CAD build for the part. Positions are in the model's coordinates, mm. A direction names the side the tool comes from. Give positions to 0.01 mm unless a question says otherwise; leave off trailing zeros. Loops run counter-clockwise (first coordinate to the right, second up) from the corner with the lowest first, then second, coordinate; pieces in that order, holes last.
Item 1: Probe probe 1 along X at (y, z) = (-4, -3); probe 2 along Z at (x, y) = (0, -1.85); probe 3 along Y at (x, z) = (11, -20). List the from-to ranges inside material, lowest first.
Item 2: Saw through at C-C on x = 7. Give the cut face in (y, z), plus the area to 3 significant figures.
Item 3: Which spindle directions (+Z, -Z, +X, -X, +Y, -Y) get a long thin tool onto all of the face, cutting with end or side? Do faces 4 (the cylindrical face through (0.31, -0.57, -21.9)), 5 (the flat face through (0, -2.5, -7)). Say none if no direction does.
Item 4: Saw through at A-A on z = -2.5. Give the cut face in (x, y).
Item 5: Drop flat-ended pins along their axis: P1, Ø8, axis at x = 10, z = 2.5, coming from the -Y side; P2, Ø1.5, axis at x = 15, y = -3, coming from the -Z side; P3, Ø0.8, axis at x = 4, y = -4, coming from the -Z side. Give the stop position or say it passes through.
Item 6: Mould opens along X. For faces 1 (the flat face through (-22.5, -3, -5)), 2 (the cylindrical face through (-4.296, -1.268, 0.189)), 3 (the flat face through (-0.31, -2.15, -22.5)) say: released by +X, released by -X, zero draft, split by the parting line, or undercut.
Item 7: Saw through at D-D on z = -12.5. Give the cut face in (x, y).
Item 8: Saw through at B-B on y = -3.25. Give the cut face in (x, z), plus the area to 3 significant figures.
from build123d import *

# Parameters (mm, degrees)
F0_W     = 45
F0_H     = 45
F1_DEPTH = 2.5
F2_SIZE  = 10.5
F4_DEPTH = 2.5
F5_R     = 2
F3_R     = 4.3
F6_DEPTH = 25
F8_DEPTH = 2


with BuildPart() as f1:
    # F0 (on Front) → F1 (new body)
    with BuildSketch(Plane.XZ):
        Rectangle(F0_W, F0_H)
    extrude(amount=F1_DEPTH)

    # F2
    f2_edges = [f1.edges().sort_by_distance(p)[0] for p in [
        (-22.5, -1.25, 22.5),
        (22.5, -1.25, 22.5),
    ]]
    chamfer(f2_edges, length=F2_SIZE)

    # F3 (on face) → F4 (join)
    with BuildSketch(Plane.XZ.offset(2.5)):
        Polygon((-17.5, -22.5), (-17.5, 9.928932), (-9.928932, 17.5), (9.928932, 17.5), (17.5, 9.928932), (17.5, -22.5), (22.5, -22.5), (22.5, 12), (12, 22.5), (-12, 22.5), (-22.5, 12), (-22.5, -22.5), align=None)
    extrude(amount=F4_DEPTH)

    # F5
    f5_edges = [f1.edges().sort_by_distance(p)[0] for p in [
        (22.5, 0, -5.25),
        (17.25, 0, 17.25),
        (0, 0, -22.5),
        (0, 0, 22.5),
        (-22.5, 0, -5.25),
        (-17.25, 0, 17.25),
    ]]
    fillet(f5_edges, radius=F5_R)

    # F3 (on face) → F6 (cut)
    with BuildSketch(Plane.XZ.offset(2.5)):
        Circle(F3_R)
    extrude(amount=-F6_DEPTH, mode=Mode.SUBTRACT)

    # F7 (on face) → F8 (join)
    with BuildSketch(Plane.XZ.offset(5)):
        with BuildLine():
            ThreePointArc((-20, 8.578932), (-19.045406, 8.974338), (-18.65, 9.928932))
            Line((-18.65, 9.928932), (-20, 9.928932))
            Line((-20, 9.928932), (-20, 8.578932))
        make_face()
        with BuildLine():
            Line((-20, 9.928932), (-18.65, 9.928932))
            ThreePointArc((-18.65, 9.928932), (-20.954594, 10.883526), (-20, 8.578932))
            Line((-20, 8.578932), (-20, 9.928932))
        make_face()
        with BuildLine():
            ThreePointArc((-21.35, -20), (-20.954594, -20.954594), (-20, -21.35))
            Line((-20, -21.35), (-20, -20))
            Line((-20, -20), (-21.35, -20))
        make_face()
        with BuildLine():
            Line((-20, -20), (-20, -21.35))
            ThreePointArc((-20, -21.35), (-19.045406, -20.954594), (-18.65, -20))
            ThreePointArc((-18.65, -20), (-20, -18.65), (-21.35, -20))
            Line((-21.35, -20), (-20, -20))
        make_face()
        with BuildLine():
            Line((20, -20), (18.65, -20))
            ThreePointArc((18.65, -20), (19.045406, -20.954594), (20, -21.35))
            Line((20, -21.35), (20, -20))
        make_face()
        with BuildLine():
            ThreePointArc((21.35, -20), (20, -18.65), (18.65, -20))
            Line((18.65, -20), (20, -20))
            Line((20, -20), (20, -21.35))
            ThreePointArc((20, -21.35), (20.954594, -20.954594), (21.35, -20))
        make_face()
        with BuildLine():
            Line((20, 9.928932), (18.65, 9.928932))
            ThreePointArc((18.65, 9.928932), (19.045406, 8.974338), (20, 8.578932))
            Line((20, 8.578932), (20, 9.928932))
        make_face()
        with BuildLine():
            ThreePointArc((21.35, 9.928932), (20, 11.278932), (18.65, 9.928932))
            Line((18.65, 9.928932), (20, 9.928932))
            Line((20, 9.928932), (20, 8.578932))
            ThreePointArc((20, 8.578932), (20.954594, 8.974338), (21.35, 9.928932))
        make_face()
        with BuildLine():
            ThreePointArc((1.35, 20), (-0.954594, 20.954594), (0, 18.65))
            ThreePointArc((0, 18.65), (0.954594, 19.045406), (1.35, 20))
        make_face()
    extrude(amount=F8_DEPTH)


solid = f1.part
Results below:
1. probe 1: x = -22.5 to -17.5, 17.5 to 22.5
1. probe 2: z = -22.49 to -4.3, 4.3 to 22.49
1. probe 3: y = -2.5 to 0
2. outline: (-5, 17.5) - (-2.5, 17.5) - (-2.5, -22.5) - (-2, -22.5) arc R2 ccw to (0, -20.5) - (0, 20.5) arc R2 ccw to (-2, 22.5) - (-5, 22.5) - close
2. area: 123 mm2
3. face 4: -Z, +X, -X, +Y
3. face 5: -Z, -Y
4. outline: (-22.5, -5) - (-17.5, -5) - (-17.5, -2.5) - (-3.5, -2.5) - (-3.5, 0) - (-20.5, 0) arc R2 ccw to (-22.5, -2) - close; (3.5, -2.5) - (17.5, -2.5) - (17.5, -5) - (22.5, -5) - (22.5, -2) arc R2 ccw to (20.5, 0) - (3.5, 0) - close
5. P1: stops at y = -2.5
5. P2: stops at z = -22.5
5. P3: stops at z = 17.5
6. face 1: released by -X
6. face 2: undercut
6. face 3: zero draft
7. outline: (-22.5, -5) - (-17.5, -5) - (-17.5, -2.5) - (17.5, -2.5) - (17.5, -5) - (22.5, -5) - (22.5, -2) arc R2 ccw to (20.5, 0) - (-20.5, 0) arc R2 ccw to (-22.5, -2) - close
8. outline: (-22.5, -22.5) - (-17.5, -22.5) - (-17.5, 9.93) - (-9.93, 17.5) - (9.93, 17.5) - (17.5, 9.93) - (17.5, -22.5) - (22.5, -22.5) - (22.5, 12) - (12, 22.5) - (-12, 22.5) - (-22.5, 12) - close
8. area: 572 mm2
